The listing builds one solid part. Answer for the finished solid, in the listing's coordinates (mm). Face numbers are marked on the shaded views. Round coordinates to 2 decimals unless told otherwise and drop trailing zeros. Write each loop counter-clockwise with the first axis right and the second up, starting at its lowest first coordinate (ties: lowest second). Pieces come first, ordered by that corner, then holes. Notation, with made-up numbers: (68.25, 49.25) - (87.25, 49.25) arc R18 cw to (87.25, 62.25) - close; hole circle Ø4 at (89, 57.5). An arc over 180 degrees is marked (long way). Answer in a Markdown table with one row per item.
from build123d import *
from build123d.topology import SkipClean

# Parameters (mm, degrees)
SKETCH1_R               = 50
BOSS_EXTRUDE1_DEPTH     = 6
SKETCH2_R               = 4.999999999999999
BOSS_EXTRUDE2_DEPTH     = 5
SKETCH3_R               = 3
CUT_EXTRUDE1_DEPTH      = 72.56116265125938
CUT_EXTRUDE2_DEPTH      = 71.96477999684069
CUT_EXTRUDE2_DEPTH_BACK = 31
SKETCH4_R               = 50
CHAMFER1_SIZE           = 0.5


with BuildPart() as part:
    # Sketch1 → Boss-Extrude1 (new body)
    with BuildSketch(Plane.XY):
        Circle(SKETCH1_R)
    extrude(amount=BOSS_EXTRUDE1_DEPTH)

    # Sketch2 → Boss-Extrude2 (add)
    with BuildSketch(Plane.XY.offset(6)):
        with Locations((0, 38)):
            Circle(SKETCH2_R)
        with BuildLine():
            ThreePointArc((-20.589119557081666, 14.180555555555557), (-4.59e-15, -25.000000000000007), (20.589119557081666, 14.180555555555557))
            ThreePointArc((20.589119557081666, 14.180555555555557), (-4.82e-15, 5.9999999999999964), (-20.589119557081666, 14.180555555555557))
        make_face()
    extrude(amount=BOSS_EXTRUDE2_DEPTH)

    # Sketch3 → Cut-Extrude1 (cut, through all)
    with BuildSketch(Plane.XY.offset(11)):
        Circle(SKETCH3_R)
    extrude(amount=-CUT_EXTRUDE1_DEPTH, mode=Mode.SUBTRACT)

    # Sketch4 → Cut-Extrude2 (cut, two sides: drawn at the far end of the back side and taken through both)
    with SkipClean():  # the faces are left unmerged after this step: merging them gives an invalid solid
        with BuildSketch(Plane.XY.offset(6).offset(-CUT_EXTRUDE2_DEPTH_BACK)):
            Circle(SKETCH4_R)
            with BuildLine():
                ThreePointArc((20.58911955708167, 14.180555555555559), (8.9e-16, -25.000000000000014), (-20.58911955708167, 14.180555555555559))
                Line((-20.589119557081666, 14.180555555555562), (-4.992793047790904, 38.268360917297514))
                ThreePointArc((-4.9927930477907125, 38.268360917297436), (-4.1970479921117985, 40.71749667008265), (-2.2879979935196513, 42.44579185091363))
                ThreePointArc((-2.2879979935196513, 42.44579185091363), (-4.1769426665e-07, 42.999999999999986), (2.287997250726913, 42.44579223318703))
                ThreePointArc((2.287997250726913, 42.44579223318703), (4.1970479585600895, 40.71749672190172), (4.992793086001126, 38.26836020640056))
                Line((4.992793086001273, 38.268360206400615), (20.58911955708167, 14.180555555555559))
            make_face(mode=Mode.SUBTRACT)
        extrude(amount=CUT_EXTRUDE2_DEPTH + CUT_EXTRUDE2_DEPTH_BACK, mode=Mode.SUBTRACT)

    # Chamfer1
    chamfer1_edges = [part.edges().sort_by_distance(p)[0] for p in [
        (-3, 3.7e-16, 0),
        (-3, 3.7e-16, 11),
    ]]
    chamfer(chamfer1_edges, length=CHAMFER1_SIZE)


solid = part.part
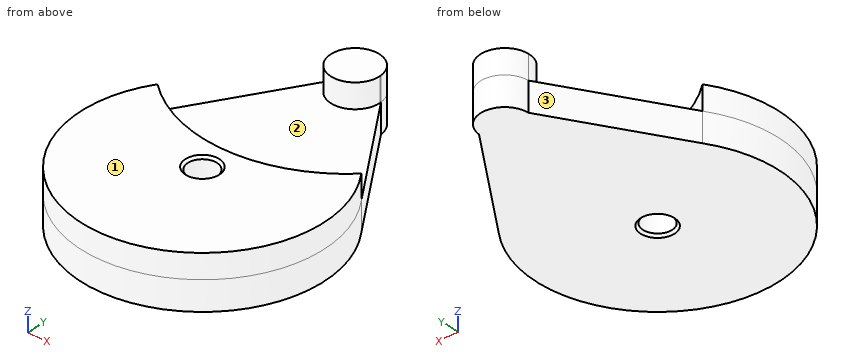
(1) Section C-C (z = 8) is taken. Give the vertices of the cut face in (x, y).
Checked values:
| item | result |
|---|---|
| outline | (-20.59, 14.18) arc R25 ccw (long way) to (20.59, 14.18) arc R30 cw to start; circle Ø10 at (0, 38); hole circle Ø6 at (0, 0) |
(2) Section B-B (x = 0) is taken. Give the vertices of the cut face in (y, z), and give its area (4 significant figures).
Checked values:
| item | result |
|---|---|
| outline | (-25, 0) - (-3.5, 0) - (-3, 0.5) - (-3, 10.5) - (-3.5, 11) - (-25, 11) - close; (3, 0.5) - (3.5, 0) - (43, 0) - (43, 11) - (33, 11) - (33, 6) - (6, 6) - (6, 11) - (3.5, 11) - (3, 10.5) - close |
| area | 546.5 mm2 |
(3) Flat-ended cylindrical pins translate along their axes: pin 1 (4 mm diameter, centred on x = 1.5, z = 5, fed in from +Y); pin 2 (3.5 mm diameter, centred on x = 0, y = 0, fed in from +Z); pin 3 (5 mm diameter, centred on x = -20, z = 9.5, fed in from +Y); pin 4 (4 mm diameter, centred on y = 20.5, z = 7, fed in from -X). Find the tip coordinate at first contact, or state that the pin passes through.
Checked values:
| item | result |
|---|---|
| pin 1 | stops at y = 43 |
| pin 2 | passes through |
| pin 3 | stops at y = 14.18 |
| pin 4 | stops at x = -17.62 |
(4) Section A-A (y = 0) is taken. Give the vertices of the cut face in (x, z), and give its area (4 significant figures).
Checked values:
| item | result |
|---|---|
| outline | (-25, 0) - (-3.5, 0) - (-3, 0.5) - (-3, 10.5) - (-3.5, 11) - (-25, 11) - close; (3, 0.5) - (3.5, 0) - (25, 0) - (25, 11) - (3.5, 11) - (3, 10.5) - close |
| area | 483.5 mm2 |
(5) For a pull along X with two mould halves and no side action, classify the marked faces 1, 2 and 3 as pulls with the +X half, pulls with the -X half, needs draft (parallel to the pull), parting line crosses it, or undercut.
Checked values:
| item | result |
|---|---|
| face 1 | needs draft |
| face 2 | undercut |
| face 3 | pulls with the -X half |
(6) Section D-D (x = 6.5) is taken. Give the vertices of the cut face in (y, z).
Checked values:
| item | result |
|---|---|
| outline | (-24.14, 0) - (35.94, 0) - (35.94, 6) - (6.71, 6) - (6.71, 11) - (-24.14, 11) - close |
(7) Find the intervals of material crossed by line 1 (Y direction, x = -1.5, z = 1); line 2 (Y direction, x = -4, z = 9); line 3 (X direction, y = -13, z = 2.75), in increasing order.
Checked values:
| item | result |
|---|---|
| line 1 | y = -24.95 to -2.6, 2.6 to 42.77 |
| line 2 | y = -24.68 to 6.27, 35 to 41 |
| line 3 | x = -21.35 to 21.35 |
